from build123d import *

# Parameters (mm, degrees)
BOSS_EXTRUDE1_DEPTH = 2
FILLET1_R           = 1
SKETCH4_W           = 17.3
SKETCH4_H           = 17.7
CUT_EXTRUDE3_DEPTH  = 1
BOSS_EXTRUDE3_REACH = 26.784
CUT_EXTRUDE5_REACH  = 21.144
SKETCH7_W           = 6.5
SKETCH7_H           = 3
CUT_EXTRUDE6_DEPTH  = 3.5
FILLET3_R           = 0.5
BOSS_EXTRUDE4_DEPTH = 20
SKETCH10_R          = 2.5
CUT_EXTRUDE7_DEPTH  = 1
FILLET4_R           = 2


# Some blends are built 0.0001 mm under size
with BuildPart() as part:
    # Sketch1 → Boss-Extrude1 (new body)
    with BuildSketch(Plane(origin=(0, 0, 0), x_dir=(1, 0, 0), z_dir=(0, 1, 0))):
        Polygon((10, -11.5), (10, 11.5), (8, 11.5), (8, 14.5), (4, 14.5), (4, 11.5), (3.25, 11.5), (3.25, 3.5), (-3.25, 3.5), (-3.25, 11.5), (-4, 11.5), (-4, 14.5), (-8, 14.5), (-8, 11.5), (-10, 11.5), (-10, -11.5), align=None)
    extrude(amount=BOSS_EXTRUDE1_DEPTH)

    # Fillet1
    fillet1_edges = [part.edges().sort_by_distance(p)[0] for p in [
        (-3.25, 1, -3.5),
        (3.25, 1, -3.5),
        (-8, 0, -13),
        (-8, 2, -13),
        (4, 0, -13),
        (4, 2, -13),
        (8, 0, -13),
        (8, 2, -13),
        (-4, 0, -13),
        (-4, 2, -13),
    ]]
    fillet(fillet1_edges, radius=FILLET1_R - 0.0001)  # a hair under: the kernel refuses the full size

    # Sketch4 → Cut-Extrude3 (cut)
    with BuildSketch(Plane(origin=(0, 2, 0), x_dir=(1, 0, 0), z_dir=(0, 1, 0))):
        with Locations((0, -0.65)):
            Rectangle(SKETCH4_W, SKETCH4_H)
    extrude(amount=-CUT_EXTRUDE3_DEPTH, mode=Mode.SUBTRACT)

    # Boss-Extrude3: up to this face of the body (flat: up to its plane)
    boss_extrude3_end = Plane(part.part.faces().sort_by_distance((-10, 1, 0))[0])
    # Sketch5 → Boss-Extrude3 (add, up to the picked face)
    with BuildSketch(Plane(origin=(10, 0, 0), x_dir=(0, 0, -1), z_dir=(1, 0, 0)), mode=Mode.PRIVATE) as boss_extrude3_sk1:
        Polygon((-11.5, 2), (-9.5, 2), (-9.5, 6.3), (-8.75, 6.3), (-8.75, 7.5), (-11.5, 7.5), align=None)
    boss_extrude3_tool1 = split(extrude(boss_extrude3_sk1.sketch, amount=-BOSS_EXTRUDE3_REACH, mode=Mode.PRIVATE), bisect_by=boss_extrude3_end, keep=Keep.BOTH, mode=Mode.PRIVATE)
    # Sketch5 → Boss-Extrude3 (add, up to the picked face)
    with BuildSketch(Plane(origin=(10, 0, 0), x_dir=(0, 0, -1), z_dir=(1, 0, 0)), mode=Mode.PRIVATE) as boss_extrude3_sk2:
        Polygon((9, 2), (11.5, 2), (11.5, 7.5), (8.5, 7.5), (8.5, 6.3), (9, 6.3), align=None)
    boss_extrude3_tool2 = split(extrude(boss_extrude3_sk2.sketch, amount=-BOSS_EXTRUDE3_REACH, mode=Mode.PRIVATE), bisect_by=boss_extrude3_end, keep=Keep.BOTH, mode=Mode.PRIVATE)
    add(boss_extrude3_tool1.solids().sort_by(Axis((10, 4.912605, 10.396008), (-1, 0, 0)))[0])
    add(boss_extrude3_tool2.solids().sort_by(Axis((10, 4.839895, -10.187282), (-1, 0, 0)))[0])

    # Sketch7 → Cut-Extrude5 (cut, up to next)
    with BuildSketch(Plane(origin=(0, 7.5, 0), x_dir=(1, 0, 0), z_dir=(0, 1, 0)), mode=Mode.PRIVATE) as cut_extrude5_sk1:
        with Locations((0, 10)):
            Rectangle(SKETCH7_W, SKETCH7_H)
    cut_extrude5_tool1 = extrude(cut_extrude5_sk1.sketch, amount=-CUT_EXTRUDE5_REACH, mode=Mode.PRIVATE) & part.part
    add(cut_extrude5_tool1.solids().sort_by_distance((0, 7.5, -10))[0], mode=Mode.SUBTRACT)

    # Sketch8 → Cut-Extrude6 (cut)
    with BuildSketch(Plane(origin=(0, 0, -11.5), x_dir=(-1, 0, 0), z_dir=(0, 0, -1))):
        Polygon((-8.575128869, 4.2), (-9.787564435, 6.3), (-12.212435565, 6.3), (-13.424871131, 4.2), (-12.212435565, 2.1), (-9.787564435, 2.1), align=None)
        Polygon((12.212435565, 2.1), (9.787564435, 2.1), (8.575128869, 4.2), (9.787564435, 6.3), (12.212435565, 6.3), (13.424871131, 4.2), align=None)
    extrude(amount=-CUT_EXTRUDE6_DEPTH, mode=Mode.SUBTRACT)

    # Fillet3
    # the kernel refuses this fillet: 0.5 mm, written as the material it adds along each edge
    with BuildSketch(Plane(origin=(10, 6.3, 9.5), x_dir=(0, -1, 0), z_dir=(-1, 0, 0))) as fillet3_piece_1:
        with BuildLine():
            CenterArc((FILLET3_R, -FILLET3_R), FILLET3_R, 90, 90)
            Line((0, -FILLET3_R), (0, 0))
            Line((0, 0), (FILLET3_R, 0))
        make_face()
    extrude(amount=20)
    with BuildSketch(Plane(origin=(11.037564435, 6.3, -9), x_dir=(0, -1, 0), z_dir=(-1, 0, 0))) as fillet3_piece_2_section:
        with BuildLine():
            CenterArc((FILLET3_R, FILLET3_R), FILLET3_R, 180, 90)
            Line((0, FILLET3_R), (0, 0))
            Line((0, 0), (FILLET3_R, 0))
        make_face()
    fillet3_piece_2 = extrude(amount=7.787564435, mode=Mode.PRIVATE)
    fillet3_piece_2 = split(fillet3_piece_2, bisect_by=Plane(origin=(8.913707181, 4.786434839, -8.886190127), z_dir=(-0.8660254037844385, 0.5000000000000003, 0)), keep=Keep.TOP, mode=Mode.PRIVATE)
    add(fillet3_piece_2)
    with BuildSketch(Plane(origin=(-3.25, 6.3, -9), x_dir=(0, -1, 0), z_dir=(-1, 0, 0))) as fillet3_piece_3_section:
        with BuildLine():
            CenterArc((FILLET3_R, FILLET3_R), FILLET3_R, 180, 90)
            Line((0, FILLET3_R), (0, 0))
            Line((0, 0), (FILLET3_R, 0))
        make_face()
    fillet3_piece_3 = extrude(amount=7.787564435, mode=Mode.PRIVATE)
    fillet3_piece_3 = split(fillet3_piece_3, bisect_by=Plane(origin=(-8.913707181, 4.786434839, -8.886190127), z_dir=(0.8660254037844393, 0.49999999999999906, 0)), keep=Keep.TOP, mode=Mode.PRIVATE)
    add(fillet3_piece_3)

    # Sketch9 → Boss-Extrude4 (add)
    with BuildSketch(Plane(origin=(10, 0, 0), x_dir=(0, 0, -1), z_dir=(1, 0, 0))):
        Polygon((-13, 6.632050808), (-11.5, 5.766025404), (-11.5, 7.5), (-13, 7.5), align=None)
        Polygon((-11.5, 0), (-11.5, 4.033974596), (-13, 3.167949192), (-13, 0), align=None)
    extrude(amount=-BOSS_EXTRUDE4_DEPTH)

    # Sketch10 → Cut-Extrude7 (cut)
    with BuildSketch(Plane(origin=(0, 2, 0), x_dir=(1, 0, 0), z_dir=(0, 1, 0))):
        with Locations((6.65, 6.5)):
            Circle(SKETCH10_R)
    extrude(amount=-CUT_EXTRUDE7_DEPTH, mode=Mode.SUBTRACT)

    # Fillet4
    fillet4_edges = [part.edges().sort_by_distance(p)[0] for p in [
        (0, 0, 13),
    ]]
    fillet(fillet4_edges, radius=FILLET4_R)


solid = part.part
Can you work these out from the model? Positions are in its coordinate system, mm. A direction names the side the tool comes from. Round coordinates to 2 decimals unless told otherwise and drop trailing zeros. Loops run counter-clockwise (first coordinate to the right, second up) from the corner with the lowest first, then second, coordinate; pieces in that order, holes last. Notation, with made-up numbers: (39.25, 29) - (86.25, 29) arc R30 ccw to (86.25, 66) - close; hole circle Ø2 at (82, 15.25). An arc over 180 degrees is marked (long way). Write item = value, one per line. Start each with the question number.
(1) If we section it at B-B (z = -9.5): Please give me the cut outline in (x, y).
(2) For faces 4 (the face through (-9.19, 3.135, -10.268)), 5 (the face through (-7, 7, -8.5)), 6 (the face through (4, 1.5, -8.2)), 7 (the face through (-4.285, 0.301, -13.021)), 8 (the face through (-9, 2, -1)), which set-ups out of +Z, -Z, +X, -X, +Y, -Y let a thin tool reach every point of the face, with its end or its side?
(3) If we section it at D-D (z = -6.25): Please give me the cut outline in (x, y), and give its area (3 significant figures).
(4) If I drill on probe 1 along Z at (x, y) = (3.75, 3); probe 2 along X at (y, z) = (1.25, 6); probe 3 along Z at (x, y) = (6, 4.75), over which ranges is the centre line in solid material (lowest first)? Write a range as [from, to].
(5) For P1, Ø0.8, axis at x = 4, y = 1.5, coming from the +Z side; P2, Ø1.1, axis at x = -5, y = 4.5, coming from the +Z side; P3, Ø5, axis at x = -4, z = 3, coming from the +Y side, each with a flat end and sliding along its axis, tell me the tip position at first contact or that it passes through.
(6) If we section it at C-C (x = -0.75): Please give me the cut outline in (y, z), and give its area (3 significant figures).
(7) If we mould it in two halves opening along Z, with no side actions, what happens to faces 1 (the face through (10, 1.5, 3.5)), 2 (the face through (0.14, 6.205, 12.26)), 3 (the face through (8.65, 1.5, 2.4))? For each: released by +Z, released by -Z, zero draft, split by the parting line, or undercut.
(8) If we section it at A-A (y = 7): Please give me the cut outline in (x, z), and give its area (4 significant figures).
Ans:
q1.outline = (-10, 0) - (-3.25, 0) - (-3.25, 7.5) - (-10, 7.5) - (-10, 6.3) - (-9.79, 6.3) - (-8.58, 4.2) - (-9.79, 2.1) - (-10, 2.1) - close; (3.25, 0) - (10, 0) - (10, 2.1) - (9.79, 2.1) - (8.58, 4.2) - (9.79, 6.3) - (10, 6.3) - (10, 7.5) - (3.25, 7.5) - close
q2.face_4 = -Z, -X
q2.face_5 = +X, -X, +Y
q2.face_6 = +Y
q2.face_7 = -Z, -Y
q2.face_8 = +X, -X
q3.outline = (-10, 0) - (-3.25, 0) - (-3.25, 1) - (-8.65, 1) - (-8.65, 2) - (-10, 2) - close; (3.25, 0) - (10, 0) - (10, 2) - (9.14, 2) - (9.14, 1) - (3.25, 1) - close
q3.area = 15.7 mm²
q4.probe_1 = [-11.5, -9], [9.5, 13]
q4.probe_2 = [-10, -8.65], [8.65, 10]
q4.probe_3 = [-11.5, -9], [9.5, 11.5]
q5.P1 = 13
q5.P2 = 11.65
q5.P3 = 1
q6.outline = (0, -3.5) - (1, -3.5) - (1, 9.5) - (5.8, 9.5) arc R0.5 cw to (6.3, 9) - (6.3, 8.75) - (7.5, 8.75) - (7.5, 13) - (6.63, 13) - (5.77, 11.5) - (4.03, 11.5) - (3.17, 13) - (2, 13) arc R2 ccw to (0, 11) - close
q6.area = 35.4 mm²
q7.face_1 = zero draft
q7.face_2 = released by +Z
q7.face_3 = undercut
q8.outline = (-10, -11.5) - (-3.25, -11.5) - (-3.25, -8.5) - (-10, -8.5) - close; (-10, 8.75) - (10, 8.75) - (10, 13) - (-10, 13) - close; (3.25, -11.5) - (10, -11.5) - (10, -8.5) - (3.25, -8.5) - close
q8.area = 125.5 mm²
